Geometry check sheet. Reference: the model listing, model coordinates, mm. A direction names the side the tool comes from. Coordinates: 2 decimals unless noted, no trailing zeros. Loops run counter-clockwise (first coordinate to the right, second up) from the corner with the lowest first, then second, coordinate; pieces in that order, holes last. Notation, with made-up numbers: M 55.5,-11 L 105.5,-11 A21 cw 105.5,10 Z; hole C -37.5,-19 d2. An arc over 180 degrees is marked long. Use CSV: the item, a comma, the result in double quotes.
```python
from build123d import *

# Parameters (mm, degrees)
SKETCH1_W             = 120
SKETCH1_H             = 20
SKETCH1_R             = 4
SKETCH1_W_2           = 35
SKETCH1_H_2           = 10
BOSS_EXTRUDE1_DEPTH   = 10
FILLET1_R             = 5
M4X0_7_TAPPED_HOLE1_D = 3.3


with BuildPart() as part:
    # Sketch1 → Boss-Extrude1 (new body)
    with BuildSketch(Plane(origin=(0, 0, 0), x_dir=(1, 0, 0), z_dir=(0, 1, 0))):
        with Locations((-60, -10)):
            Rectangle(SKETCH1_W, SKETCH1_H)
        with Locations(Location((-60, -10, 0), (0, 0, 270))):
            Circle(SKETCH1_R, mode=Mode.SUBTRACT)
        with Locations((-87.5, -10)):
            Rectangle(SKETCH1_W_2, SKETCH1_H_2, mode=Mode.SUBTRACT)
        with Locations((-32.5, -10)):
            Rectangle(SKETCH1_W_2, SKETCH1_H_2, mode=Mode.SUBTRACT)
    extrude(amount=BOSS_EXTRUDE1_DEPTH)

    # Fillet1
    fillet1_edges = [part.edges().sort_by_distance(p)[0] for p in [
        (-15, 5, 15),
        (-15, 5, 5),
        (-50, 5, 15),
        (-50, 5, 5),
        (-105, 5, 5),
        (-105, 5, 15),
        (-70, 5, 5),
        (-70, 5, 15),
    ]]
    fillet(fillet1_edges, radius=FILLET1_R - 0.0001)  # a hair under: the kernel refuses the full size

    # M4x0.7 Tapped Hole1 (through all)
    with Locations(Plane(origin=(0, 10, 0), x_dir=(1, 0, 0), z_dir=(0, 1, 0))):
        with Locations((-115, -5), (-115, -15), (-5, -5), (-5, -15)):
            Hole(M4X0_7_TAPPED_HOLE1_D / 2)


solid = part.part
```
1. Section check B-B, the plane y = 1. Count the separate pieces of the cut face and the enclosed holes in it, plus the area to 3 significant figures.
The answers:
separate pieces,"1"
enclosed holes,"7"
area,"1,660 mm^2"
2. Section check C-C, the plane x = -38. Record the cut outline in (y, z), plus the area to 3 significant figures.
The answers:
outline,"M 0,0 L 10,0 L 10,5 L 0,5 Z; M 0,15 L 10,15 L 10,20 L 0,20 Z"
area,"100 mm^2"
3. Set-up check for faces 4 (the flat face through (-120, 5, 10)), 5 (the cylindrical face through (-104, 5, 7)): record each of +Z, -Z, +X, -X, +Y, -Y from which the full face is reachable in a straight line by a thin tool's end or side.
The answers:
face 4,"+Z, -Z, -X, +Y, -Y"
face 5,"+Y, -Y"
4. Section check D-D, the plane z = 12. Record the cut outline in (x, y).
The answers:
outline,"M -120,0 L -104.58,0 L -104.58,10 L -120,10 Z; M -70.42,0 L -63.46,0 L -63.46,10 L -70.42,10 Z; M -56.54,0 L -49.58,0 L -49.58,10 L -56.54,10 Z; M -15.42,0 L 0,0 L 0,10 L -15.42,10 Z"
5. Section check A-A, the plane x = -115. Record the cut outline in (y, z).
The answers:
outline,"M 0,0 L 10,0 L 10,3.35 L 0,3.35 Z; M 0,6.65 L 10,6.65 L 10,13.35 L 0,13.35 Z; M 0,16.65 L 10,16.65 L 10,20 L 0,20 Z"
6. Thickness scan on line 1 (Z direction, x = -115, y = 4.25); line 2 (X direction, y = 3, z = 10); line 3 (Z direction, x = -92, y = 6.5). Record the ranges inside material, lowest first. Write a range as [from, to].
The answers:
line 1,"[0, 3.35], [6.65, 13.35], [16.65, 20]"
line 2,"[-120, -105], [-70, -64], [-56, -50], [-15, 0]"
line 3,"[0, 5], [15, 20]"
7. Release check for a two-part mould opening along Z. For faces 1 (the flat face through (-61, 0, 5)), 2 (the flat face through (-88, 5, 15)), 3 (the flat face through (-61, 5, 0)) record: +Z half, -Z half, draft (parallel to the pull), parting line (faces both ways), or undercut.
The answers:
face 1,"draft"
face 2,"undercut"
face 3,"-Z half"
